Can you work these out from the model? Positions are in its coordinate system, mm. A direction names the side the tool comes from. Give positions to 0.01 mm unless a question says otherwise; leave off trailing zeros. Loops run counter-clockwise (first coordinate to the right, second up) from the corner with the lowest first, then second, coordinate; pieces in that order, holes last.
from build123d import *

# Parameters (mm, degrees)
F1_DEPTH = 65
F2_R     = 33.47406
F3_DEPTH = 1.8
F5_START = -62.9
F4_R     = 33.47406
F4_R_2   = 32.57406
F5_DEPTH = 4
F7_START = -52.7
F6_R     = 4.1
F7_DEPTH = 12.3


with BuildPart() as f1:
    # F0 (on Top) → F1 (new body)
    with BuildSketch(Plane.XY):
        with BuildLine():
            ThreePointArc((-6.301205687, -31.1349322809), (0, -8.0552877694), (6.301205687, -31.1349322809))
            Line((6.301205687, -31.1349322809), (12.4, -31.1349322809))
            ThreePointArc((12.4, -31.1349322809), (24.8626517269, -22.4720394544), (32.2258282769, -9.2))
            Line((32.2258282769, -9.2), (27.7038375399, -5.6655561268))
            ThreePointArc((27.7038375399, -5.6655561268), (11.2552877694, 0), (27.7038375399, 5.6655561268))
            Line((27.7038375399, 5.6655561268), (32.2258282769, 9.2))
            ThreePointArc((32.2258282769, 9.2), (23.9908874936, 23.4004556666), (10, 31.9866223308))
            Line((10, 31.9866223308), (6.5516160367, 28.0101754131))
            ThreePointArc((6.5516160367, 28.0101754131), (0, 10.4552877694), (-6.5516160367, 28.0101754131))
            Line((-6.5516160367, 28.0101754131), (-10, 31.9866223308))
            ThreePointArc((-10, 31.9866223308), (-23.3602452547, 24.0300426503), (-31.6912291989, 10.9))
            Line((-31.6912291989, 10.9), (-28.2788214738, 7.5896192511))
            ThreePointArc((-28.2788214738, 7.5896192511), (-9.5552877694, 0), (-28.2788214738, -7.5896192511))
            Line((-28.2788214738, -7.5896192511), (-31.6912291989, -10.9))
            ThreePointArc((-31.6912291989, -10.9), (-24.256385637, -23.125132734), (-12.4, -31.1349322809))
            Line((-12.4, -31.1349322809), (-6.301205687, -31.1349322809))
        make_face()
    extrude(amount=-F1_DEPTH)

    # F2 (on Top) → F3 (join)
    with BuildSketch(Plane.XY):
        Circle(F2_R)
    extrude(amount=F3_DEPTH)

    # F4 (on Top) → F5 (join)
    with BuildSketch(Plane.XY.offset(F5_START)):
        Circle(F4_R)
        Circle(F4_R_2, mode=Mode.SUBTRACT)
    extrude(amount=-F5_DEPTH)

    # F6 (on Top) → F7 (cut)
    with BuildSketch(Plane.XY.offset(F7_START)):
        Circle(F6_R)
    extrude(amount=-F7_DEPTH, mode=Mode.SUBTRACT)


solid = f1.part
(1) Thinking about a two-plate mould opening in X: for faces 3 (the cylindrical face through (-0.453, -8.064, -32.045)), 4 (the flat face through (0, -33, -62.9)), 5 (the cylindrical face through (24.152, 23.234, -32.045)), which applies, pulls with the +X half, pulls with the -X half, needs draft (parallel to the pull), parting line crosses it, or undercut?
Returned:
face 3: undercut
face 4: needs draft
face 5: pulls with the +X half
(2) Suppose I cut it at C-C on z = -18.5. List the corners of the cut face in (x, y) for me.
Returned:
outline: (-31.69, -10.9) arc R33.51 ccw to (-12.4, -31.13) - (-6.3, -31.13) arc R12.4 cw (long way) to (6.3, -31.13) - (12.4, -31.13) arc R33.51 ccw to (32.23, -9.2) - (27.7, -5.67) arc R9.2 cw (long way) to (27.7, 5.67) - (32.23, 9.2) arc R33.51 ccw to (10, 31.99) - (6.55, 28.01) arc R10 cw (long way) to (-6.55, 28.01) - (-10, 31.99) arc R33.51 ccw to (-31.69, 10.9) - (-28.28, 7.59) arc R10.9 cw (long way) to (-28.28, -7.59) - close
(3) Suppose I cut it at D-D on x = -21. List the corners of the cut face in (y, z) for me.
Returned:
outline: (-26.12, -65) - (-26.07, -65) - (-26.07, -66.9) - (-24.9, -66.9) - (-24.9, -65) - (-10.89, -65) - (-10.89, 0) - (10.89, 0) - (10.89, -65) - (24.9, -65) - (24.9, -66.9) - (26.07, -66.9) - (26.07, -65) - (26.12, -65) - (26.12, 0) - (26.07, 0) - (26.07, 1.8) - (-26.07, 1.8) - (-26.07, 0) - (-26.12, 0) - close
(4) Will these pins go through, and if not, where does the flat tip stop? P1, Ø3, axis at x = -3.5, y = 2.5, coming from the -Z side; P2, Ø5, axis at x = 8.5, z = -27, coming from the -Y side; P3, Ø12, axis at y = -9, z = -37, coming from the -X side.
Returned:
P1: stops at z = -65
P2: stops at y = -31.13
P3: stops at x = -31.69
(5) Which directions (+Z, -Z, +X, -X, +Y, -Y) give clear straight access to the entire face, cutting with the end or side of a thin tool? Please do faces 1 (the cylindrical face through (-0.534, 4.065, -58.764)), 2 (the cylindrical face through (24.72, -22.63, -32.04)).
Returned:
face 1: -Z
face 2: +Z, -Z, +X, -Y
(6) Suppose I cut it at B-B on x = 0. List the corners of the cut face in (y, z) for me, plus the area to 3 significant figures.
Returned:
outline: (-33.47, -66.9) - (-32.57, -66.9) - (-32.57, -62.9) - (-33.47, -62.9) - close; (-33.47, 0) - (-8.06, 0) - (-8.06, -65) - (-4.1, -65) - (-4.1, -52.7) - (4.1, -52.7) - (4.1, -65) - (10.46, -65) - (10.46, 0) - (33.47, 0) - (33.47, 1.8) - (-33.47, 1.8) - close; (32.57, -66.9) - (33.47, -66.9) - (33.47, -62.9) - (32.57, -62.9) - close
area: 1,230 mm2
(7) Suppose I cut it at A-A on y = 0. List the corners of the cut face in (x, z) for me, plus the area to 3 significant figures.
Returned:
outline: (-33.47, -66.9) - (-32.57, -66.9) - (-32.57, -62.9) - (-33.47, -62.9) - close; (-33.47, 0) - (-9.56, 0) - (-9.56, -65) - (-4.1, -65) - (-4.1, -52.7) - (4.1, -52.7) - (4.1, -65) - (11.26, -65) - (11.26, 0) - (33.47, 0) - (33.47, 1.8) - (-33.47, 1.8) - close; (32.57, -66.9) - (33.47, -66.9) - (33.47, -62.9) - (32.57, -62.9) - close
area: 1,380 mm2
(8) Please list where these lines run through material, in increasing order: probe 1 along Y at (x, z) = (0, -64); probe 2 along Z at (x, y) = (-6, 16); probe 3 along Y at (x, z) = (0, -19.5).
Returned:
probe 1: y = -33.47 to -32.57, -8.06 to -4.1, 4.1 to 10.46, 32.57 to 33.47
probe 2: z = 0 to 1.8
probe 3: y = -8.06 to 10.46
